from build123d import *

# Parameters (mm, degrees)
F0_W     = 63
F0_H     = 77
F1_DEPTH = 2
F0_W_2   = 67
F0_H_2   = 81
F2_DEPTH = 20


with BuildPart() as f1:
    # F0 (on Top) → F1 (new body)
    with BuildSketch(Plane.XY):
        Rectangle(F0_W, F0_H)
        with BuildLine():
            ThreePointArc((-16.5, 18.5), (-15.035534, 22.035534), (-11.5, 23.5))
            Line((-11.5, 23.5), (11.5, 23.5))
            ThreePointArc((11.5, 23.5), (15.035534, 22.035534), (16.5, 18.5))
            Line((16.5, 18.5), (16.5, -18.5))
            ThreePointArc((16.5, -18.5), (15.035534, -22.035534), (11.5, -23.5))
            Line((11.5, -23.5), (-11.5, -23.5))
            ThreePointArc((-11.5, -23.5), (-15.035534, -22.035534), (-16.5, -18.5))
            Line((-16.5, -18.5), (-16.5, 18.5))
        make_face(mode=Mode.SUBTRACT)
    extrude(amount=F1_DEPTH)

    # F0 (on Top) → F2 (join)
    with BuildSketch(Plane.XY):
        Rectangle(F0_W_2, F0_H_2)
        Rectangle(F0_W, F0_H, mode=Mode.SUBTRACT)
    extrude(amount=F2_DEPTH)


solid = f1.part
The model under review builds one solid part; all positions refer to its coordinate system, in mm. A direction names the side the tool comes from. Round coordinates to 2 decimals unless told otherwise and drop trailing zeros. Write each loop counter-clockwise with the first axis right and the second up, starting at its lowest first coordinate (ties: lowest second). Pieces come first, ordered by that corner, then holes. Notation, with made-up numbers: M 26,86.25 L 75,86.25 A25 ccw 75,123.25 Z; hole C -9.75,31 d2. An arc over 180 degrees is marked long. Use a Markdown table: item, result. Add a question column.
Q1. Insertion check: pin 1 (12 mm diameter, centred on x = -5.5, y = -1.5, fed in from +Z). The pin has a flat end and moves straight along its axis. Give the tip position at first contact, or say it passes through.
Q2. We need section C-C, the plane y = -14. State the section outline as (x, z) points, plus the area to 3 significant figures.
Q3. Machinability: for faces 1 (the face through (31.5, -1, 11)), 2 (the face through (0, 23.5, 1)), 3 (the face through (0, 40.5, 10)), which of the approach directions +Z, -Z, +X, -X, +Y, -Y give a long, thin tool a straight path to every point of the face, cutting with its end or side? Answer none if there is none.
Q4. To check wall thickness, follow line 1 (X direction, y = -16, z = 3.75); line 2 (Y direction, x = 19, z = 10.25); line 3 (Y direction, x = -3, z = 1). State the ranges of each line that lie inside material, in increasing order.
Q5. We need section B-B, the plane x = -2. State the section outline as (y, z) points, plus the area to 3 significant figures.
Q6. We need section A-A, the plane z = 7.5. State the section outline as (x, y) points, plus the area to 3 significant figures.
Q7. The part is to be moulded in two halves that separate along X. For faces 4 (the face through (-23, 1, 0)), 5 (the face through (33.5, -1, 10)), 6 (the face through (-15.07, 22, 0.99)), say which applies: pulls with the +X half, pulls with the -X half, needs draft (parallel to the pull), parting line crosses it, or undercut.
Q8. We need section D-D, the plane y = 27. State the section outline as (x, z) points, plus the area to 3 significant figures.
Findings below:
| question | item | result |
|---|---|---|
| 1 | pin 1 | passes through |
| 2 | outline | M -33.5,0 L -16.5,0 L -16.5,2 L -31.5,2 L -31.5,20 L -33.5,20 Z; M 16.5,0 L 33.5,0 L 33.5,20 L 31.5,20 L 31.5,2 L 16.5,2 Z |
| 2 | area | 140 mm² |
| 3 | face 1 | +Z |
| 3 | face 2 | +Z, -Z |
| 3 | face 3 | +Z, -Z, +X, -X, +Y |
| 4 | line 1 | x = -33.5 to -31.5, 31.5 to 33.5 |
| 4 | line 2 | y = -40.5 to -38.5, 38.5 to 40.5 |
| 4 | line 3 | y = -40.5 to -23.5, 23.5 to 40.5 |
| 5 | outline | M -40.5,0 L -23.5,0 L -23.5,2 L -38.5,2 L -38.5,20 L -40.5,20 Z; M 23.5,0 L 40.5,0 L 40.5,20 L 38.5,20 L 38.5,2 L 23.5,2 Z |
| 5 | area | 140 mm² |
| 6 | outline | M -33.5,-40.5 L 33.5,-40.5 L 33.5,40.5 L -33.5,40.5 Z; hole M -31.5,-38.5 L 31.5,-38.5 L 31.5,38.5 L -31.5,38.5 Z |
| 6 | area | 576 mm² |
| 7 | face 4 | needs draft |
| 7 | face 5 | pulls with the +X half |
| 7 | face 6 | undercut |
| 8 | outline | M -33.5,0 L 33.5,0 L 33.5,20 L 31.5,20 L 31.5,2 L -31.5,2 L -31.5,20 L -33.5,20 Z |
| 8 | area | 206 mm² |
